Geometry check sheet. Reference: drawing and pictorial views, mm from the part's lowest x, y, z. A direction names the side the tool comes from. Give positions to 0.01 mm unless a question says otherwise; leave off trailing zeros. Order: outer loops, then holes, each group sorted by start corner. A loop starts at its lowest first (then second) coordinate and runs counter-clockwise, first axis right, second up.
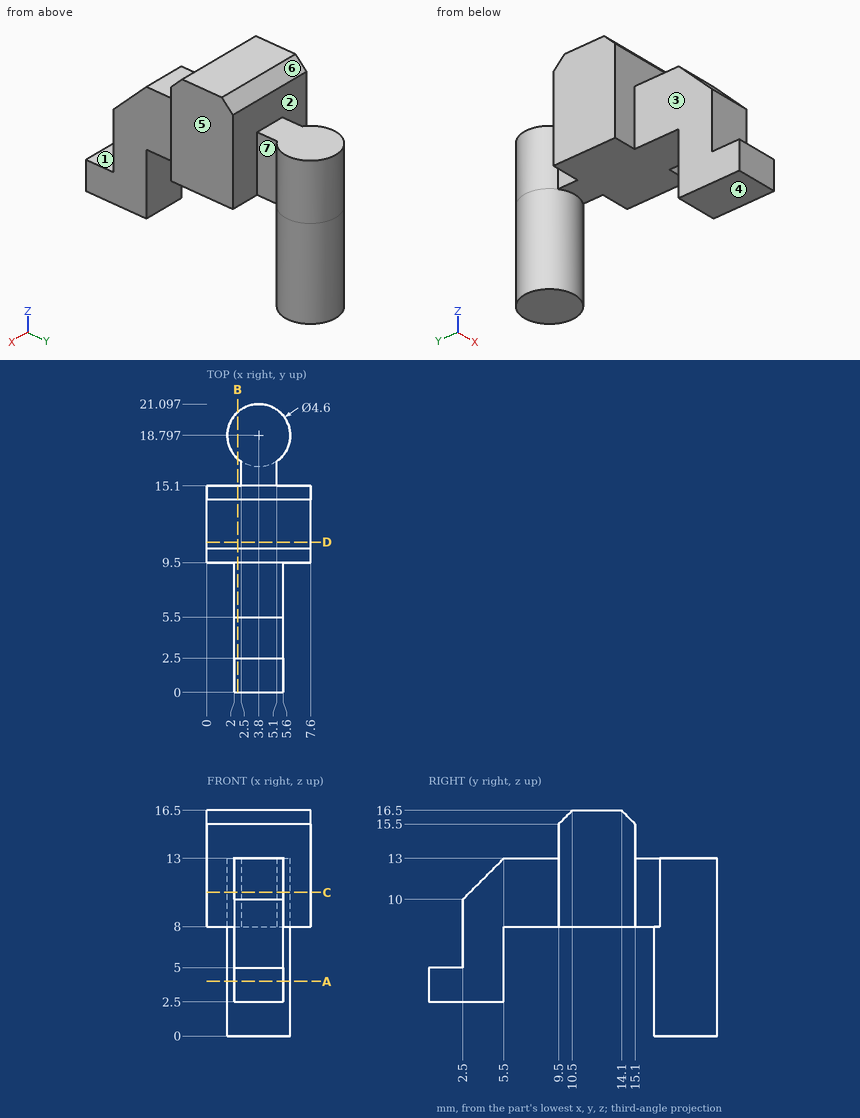
1) Section check D-D, the plane y = 11. Record the cut outline in (x, z), then the cut area to 3 significant figures.
Recorded:
outline: (0, 8) - (7.6, 8) - (7.6, 16.5) - (0, 16.5) - close
area: 64.6 mm2
2) Section check C-C, the plane z = 10.5. Record the cut outline in (x, y).
Recorded:
outline: (0, 9.5) - (2, 9.5) - (2, 3) - (5.6, 3) - (5.6, 9.5) - (7.6, 9.5) - (7.6, 15.1) - (5.1, 15.1) - (5.1, 16.9) arc R2.3 ccw (long way) to (2.5, 16.9) - (2.5, 15.1) - (0, 15.1) - close
3) Section check A-A, the plane z = 4. Record the cut outline in (x, y).
Recorded:
outline: circle Ø4.6 at (3.8, 18.8); (2, 0) - (5.6, 0) - (5.6, 5.5) - (2, 5.5) - close
4) Set-up check for the marked faces 1, 2, 3 and 4: record each of +Z, -Z, +X, -X, +Y, -Y from which the full face is reachable in a straight line by a thin tool's end or side.
Recorded:
face 1: +Z, +X, -X, -Y
face 2: +Z
face 3: +Z, -Z, -X, -Y
face 4: -Z, +X, -X, -Y
5) Draft check along Y on the marked faces 5, 6 and 7. Enter one of: +Y half, -Y half, draft (parallel to the pull), parting line (faces both ways), or undercut.
Recorded:
face 5: draft
face 6: +Y half
face 7: undercut
6) Section check B-B, the plane x = 2.25. Record the cut outline in (y, z), then the cut area to 3 significant figures.
Recorded:
outline: (0, 2.5) - (5.5, 2.5) - (5.5, 8) - (15.1, 8) - (15.1, 15.5) - (14.1, 16.5) - (10.5, 16.5) - (9.5, 15.5) - (9.5, 13) - (5.5, 13) - (2.5, 10) - (2.5, 5) - (0, 5) - close; (17.1, 0) - (20.5, 0) - (20.5, 13) - (17.1, 13) - close
area: 144 mm2
7) Material ranges on L1, parallel to Y at x = 3.75, z = 7; L2, parallel to Z at x = 2.75, y = 17.5; L3, parallel to Z at x = 5, y = 13, recorded low to high.
Recorded:
L1: y = 2.5 to 5.5, 16.5 to 21.1
L2: z = 0 to 13
L3: z = 8 to 16.5
8) Depth check by flat-ended pin: pin 1 Ø1.2 at (x, y) = (4, 1) entering from +Z; pin 2 Ø4 at (y, z) = (7, 13) entering from +X; pin 3 Ø2.5 at (x, y) = (3.5, 19.5) entering from +Z. Enter the tip coordinate at first touch or a pass-through.
Recorded:
pin 1: stops at z = 5
pin 2: stops at x = 5.6
pin 3: stops at z = 13
